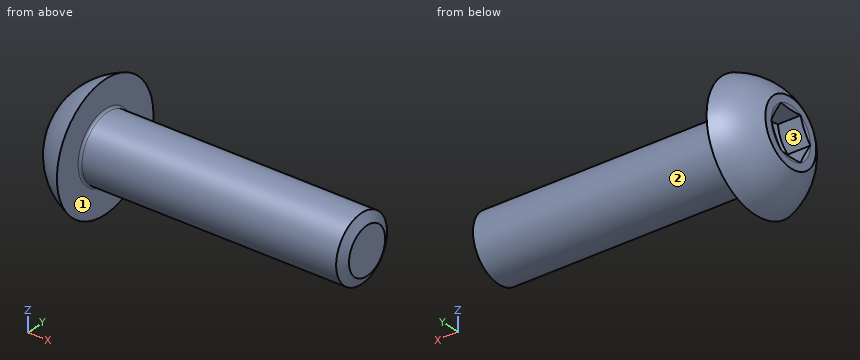
```python
from build123d import *

# Parameters (mm, degrees)
CUT_EXTRUDE_1_DEPTH = 1.65


with BuildPart() as part:
    # 草图1 → 旋转1 (revolve)
    with BuildSketch(Plane.XY):
        with BuildLine():
            Line((0, 1.5), (-11.9, 1.5))
            ThreePointArc((-11.9, 1.5), (-11.970710678, 1.529289322), (-12, 1.6))
            Line((-12, 1.6), (-12, 2.85))
            ThreePointArc((-12, 2.85), (-12.948716751, 2.326209363), (-13.65, 1.5))
            Line((-13.65, 1.5), (-13.65, 0))
            Line((-13.65, 0), (0, 0))
            Line((0, 0), (0, 1.5))
        make_face()
    revolve(axis=Axis((-13.65, 0, 0), (1, 0, 0)))

    # 草图2 → 切除-拉伸1 (cut)
    with BuildSketch(Plane.ZY.offset(13.65)):
        Polygon((0, 1.154700538), (-1, 0.577350269), (-1, -0.577350269), (0, -1.154700538), (1, -0.577350269), (1, 0.577350269), align=None)
    extrude(amount=-CUT_EXTRUDE_1_DEPTH, mode=Mode.SUBTRACT)

    # 草图6 → 旋转2 (revolve)
    with BuildSketch(Plane.XY):
        Polygon((-12.61, 1.154700538), (-12, 0), (-11.7, 0), (-11.7, 1.154700538), align=None)
    revolve(axis=Axis((-13.65, 0, 0), (1, 0, 0)))

    # 草图7 → 切除-旋转5 (revolve, cut)
    with BuildSketch(Plane.XY):
        Polygon((-13.65, 1.154700538), (-13.35, 0), (-13.65, 0), align=None)
    revolve(axis=Axis((-13.65, 0, 0), (1, 0, 0)), mode=Mode.SUBTRACT)

    # 草图4 → 切除-旋转1 (revolve, cut)
    with BuildSketch(Plane.XY):
        Polygon((-0.25, 1.5), (0, 1.066987298), (0.25, 1.5), align=None)
    revolve(axis=Axis((-0.25, 0, 0), (1, 0, 0)), mode=Mode.SUBTRACT)


solid = part.part
```
Input: part model. Units: mm. Frame: model coordinates. Face numbers are marked on the shaded views. Give positions to 0.01 mm unless a question says otherwise; leave off trailing zeros. Order: outer loops, then holes, each group sorted by start corner. A loop starts at its lowest first (then second) coordinate and runs counter-clockwise, first axis right, second up. Notation, with made-up numbers: (49.5, 56) - (103.5, 56) arc R11 ccw to (103.5, 61) - close; hole circle Ø5 at (53, 68). An arc over 180 degrees is marked (long way). Use a Markdown table: item, result.
(1) Pin query (flat end, axial travel): pin 1 (1 mm diameter, centred on x = -2.5, z = -1.5, fed in from +Y); pin 2 (1 mm diameter, centred on x = -5.5, z = -0.5, fed in from -Y); pin 3 (0.9 mm diameter, centred on x = -13.5, y = 0, fed in from +Z); pin 4 (3 mm diameter, centred on y = -0.5, z = -0.5, fed in from +X). Return the tip coordinate at first contact, or that it passes through.
Computed values:
| item | result |
|---|---|
| pin 1 | stops at y = 1.12 |
| pin 2 | stops at y = -1.5 |
| pin 3 | stops at z = 2.24 |
| pin 4 | stops at x = 0 |
(2) Section query B-B (z = -2.4). Output: boundary loops of the cut face in (x, y), then the cut area to 3 significant figures.
Computed values:
| item | result |
|---|---|
| outline | (-12, -1.54) - (-12, 1.54) arc R1.81 ccw to start |
| area | 1.86 mm2 |
(3) Line query: line 1 (Z direction, x = -13, y = -1.1); line 2 (X direction, y = -2, z = -1.95); line 3 (Y direction, x = -1, z = 0.65). Output: solid intervals per line, ascending. Write a range as from..to.
Computed values:
| item | result |
|---|---|
| line 1 | z = -2..-0.09, 0.09..2 |
| line 2 | x = -12.16..-12 |
| line 3 | y = -1.35..1.35 |
(4) Section query C-C (y = 1.75). Output: boundary loops of the cut face in (x, z), then the cut area to 3 significant figures.
Computed values:
| item | result |
|---|---|
| outline | (-12, -2.25) - (-12, 2.25) arc R2.44 ccw to start |
| area | 4.84 mm2 |
(5) Draft query along Z for the marked faces 1, 2 and 3. Return one class per face: released by +Z, released by -Z, zero draft, split by the parting line, or undercut.
Computed values:
| item | result |
|---|---|
| face 1 | zero draft |
| face 2 | split by the parting line |
| face 3 | undercut |
(6) Section query A-A (x = -1.5). Output: boundary loops of the cut face in (y, z), then the cut area to 3 significant figures.
Computed values:
| item | result |
|---|---|
| outline | circle Ø3 at (0, 0) |
| area | 7.07 mm2 |
